```python
from build123d import *

# Parameters (mm, degrees)
BOSS_EXTRUDE1_DEPTH      = 1.5
BOSS_EXTRUDE1_DEPTH_BACK = 1.2
CUT_EXTRUDE1_DEPTH       = 40
FILLET1_R                = 1


with BuildPart() as part:
    # Sketch1 → Boss-Extrude1 (new body, two sides)
    with BuildSketch(Plane.XY) as boss_extrude1_sk:
        with BuildLine():
            Line((-17.999999991, 9.304537824), (-17.999999991, 10.304506021))
            Line((-17.999999991, 10.304506021), (-17.999999991, 17.303464443))
            ThreePointArc((-17.999999991, 17.303464443), (-17.707106772, 18.010571225), (-16.999999991, 18.303464443))
            Line((-16.999999991, 18.303464443), (16.999968161, 18.303464443))
            ThreePointArc((16.999968161, 18.303464443), (17.707074942, 18.010571225), (17.999968161, 17.303464443))
            Line((17.999968161, 17.303464443), (17.999968161, 9.303464443))
            Line((17.999968161, 9.303464443), (17.999968161, 6.751174458))
            ThreePointArc((17.999968161, 6.751174458), (17.707074942, 6.044067677), (16.999968161, 5.751174458))
            Line((16.999968161, 5.751174458), (16.499999991, 5.751174458))
            ThreePointArc((16.499999991, 5.751174458), (16.1464466, 5.604727849), (15.999999991, 5.251174458))
            Line((15.999999991, 5.251174458), (15.999999991, 2.751174458))
            ThreePointArc((15.999999991, 2.751174458), (15.707106772, 2.044067677), (14.999999991, 1.751174458))
            Line((14.999999991, 1.751174458), (-14.999999991, 1.751174458))
            ThreePointArc((-14.999999991, 1.751174458), (-15.707106772, 2.044067677), (-15.999999991, 2.751174458))
            Line((-15.999999991, 2.751174458), (-15.999999991, 5.251174458))
            ThreePointArc((-15.999999991, 5.251174458), (-16.1464466, 5.604727849), (-16.499999991, 5.751174458))
            Line((-16.499999991, 5.751174458), (-16.999999991, 5.751174458))
            ThreePointArc((-16.999999991, 5.751174458), (-17.707106772, 6.044067677), (-17.999999991, 6.751174458))
            Line((-17.999999991, 6.751174458), (-17.999999991, 9.304537824))
        make_face()
    extrude(amount=BOSS_EXTRUDE1_DEPTH)
    extrude(boss_extrude1_sk.sketch, amount=-BOSS_EXTRUDE1_DEPTH_BACK)

    # Sketch3 → Cut-Extrude1 (cut)
    with BuildSketch(Plane(origin=(17.999968161, 0, 0), x_dir=(0, 0, -1), z_dir=(1, 0, 0))):
        with BuildLine():
            Line((0.023796664, 5.754537824), (0.023796664, 10.304537824))
            Line((0.023796664, 10.304537824), (1.023796664, 10.304537824))
            Line((1.023796664, 10.304537824), (1.023796664, 22.680762846))
            ThreePointArc((1.023796664, 22.680762846), (7.212872074, 16.614024598), (1.2708887, 10.304537824))
            Line((1.2708887, 10.304537824), (1.2708887, 1.751174458))
            Line((1.2708887, 1.751174458), (0.23729316, 1.751174458))
            ThreePointArc((0.23729316, 1.751174458), (0.053060483, 3.748723952), (0.023796664, 5.754537824))
        make_face()
        with BuildLine():
            Line((-1.5, 3.645881873), (-1.5, 1.751174458))
            Line((-1.5, 1.751174458), (-0.306090164, 1.751174458))
            Line((-0.306090164, 1.751174458), (-0.348355137, 1.751174458))
            ThreePointArc((-0.348355137, 1.751174458), (-0.398355137, 1.764571918), (-0.434957677, 1.801174458))
            Line((-0.434957677, 1.801174458), (-1.5, 3.645881873))
        make_face()
    extrude(amount=-CUT_EXTRUDE1_DEPTH, mode=Mode.SUBTRACT)

    # Fillet1
    fillet1_edges = [part.edges().sort_by_distance(p)[0] for p in [
        (0, 3.645881873, 1.5),
    ]]
    fillet(fillet1_edges, radius=FILLET1_R)


solid = part.part
```
Source: CAD feature listing. Evaluate the final solid. Frame: model axes, mm. A direction names the side the tool comes from. Give positions to 0.01 mm unless a question says otherwise; leave off trailing zeros. Loops run counter-clockwise (first coordinate to the right, second up) from the corner with the lowest first, then second, coordinate; pieces in that order, holes last. Notation, with made-up numbers: (-22.75, 59) -> (35.25, 59) arc R22 cw to (35.25, 80) -> close; hole circle Ø7 at (51, -6.5). An arc over 180 degrees is marked (long way). Put each result on its own line as item: value. Start each with the question number.
1) Cut plane C-C (y = 7.75). Return loops of the section in (x, z).
2) Cut plane A-A (x = -1). Return loops of the section in (y, z).
3) Cut plane B-B (z = -0.65). Return loops of the section in (x, y).
4) Material intervals for probe 1 along Z at (x, y) = (4, 9); probe 2 along Y at (x, z) = (16.5, 0.9); probe 3 along Z at (x, y) = (-9.5, 2.75), sorted ascending.
5) Contact query for flat-ended pins moving along their axis: P1, Ø1.5, axis at y = 6.5, z = 1, coming from the -X side; P2, Ø0.8, axis at y = 4, z = 0.5, coming from the +X side; P3, Ø0.5, axis at y = 4, z = 0.5, coming from the -X side. Output: stop coordinate, or through.
6) Draft query along Y for faces 4 (the face through (0.3, 10.305, -0.5)), 5 (the face through (-16, 4, 1)), 6 (the face through (-15.813, 2.169, 0.246)). Return one class per face: released by +Y, released by -Y, zero draft, split by the parting line, or undercut.
7) Reachability of faces 1 (the face through (0.224, 2.596, 0.894)), 2 (the face through (0, 8, -0.024)), 3 (the face through (16, 4, 1)) from +Z, -Z, +X, -X, +Y, -Y: full face, straight path, thin tool, end or side. Return the list, or none.
Results are:
1. outline: (-18, -0.02) -> (18, -0.02) -> (18, 1.5) -> (-18, 1.5) -> close
2. outline: (1.75, -0.24) arc R25.93 cw to (5.75, -0.02) -> (10.3, -0.02) -> (10.3, -1.02) -> (18.3, -1.02) -> (18.3, 1.5) -> (3.91, 1.5) arc R1 ccw to (3.41, 1.37) -> (1.8, 0.43) arc R0.1 ccw to (1.75, 0.35) -> close
3. outline: (-18, 10.3) -> (18, 10.3) -> (18, 17.3) arc R1 ccw to (17, 18.3) -> (-17, 18.3) arc R1 ccw to (-18, 17.3) -> close
4. probe 1: z = -0.02 to 1.5
4. probe 2: y = 5.75 to 18.3
4. probe 3: z = -0.13 to 0.98
5. P1: stops at x = -18
5. P2: stops at x = 16
5. P3: stops at x = -16
6. face 4: undercut
6. face 5: zero draft
6. face 6: released by -Y
7. face 1: +Z, +X, -X, -Y
7. face 2: -Z, +X, -X
7. face 3: +Z, -Z, +X, -Y
